from build123d import *

# Parameters (mm, degrees)
IZIM1_R                     = 15
Y_KSEKLIK_EKSTR_ZYON1_DEPTH = 55
IZIM2_R                     = 25
Y_KSEKLIK_EKSTR_ZYON2_DEPTH = 25
IZIM3_R                     = 30
Y_KSEKLIK_EKSTR_ZYON3_DEPTH = 20
IZIM4_W                     = 21.622627276
IZIM4_H                     = 20
KES_EKSTR_ZYON1_DEPTH       = 20
IZIM6_R                     = 4
KES_EKSTR_ZYON2_DEPTH       = 30
KES_EKSTR_ZYON3_DEPTH       = 30


with BuildPart() as part:
    # Çizim1 → Yükseklik-Ekstrüzyon1 (new body)
    with BuildSketch(Plane.XY):
        Circle(IZIM1_R)
    extrude(amount=-Y_KSEKLIK_EKSTR_ZYON1_DEPTH)

    # Çizim2 → Yükseklik-Ekstrüzyon2 (add)
    with BuildSketch(Plane(origin=(0, 0, -55), x_dir=(-1, 0, 0), z_dir=(0, 0, -1))):
        with Locations(Location((0, 10, 0), (0, 0, 270))):
            Circle(IZIM2_R)
    extrude(amount=Y_KSEKLIK_EKSTR_ZYON2_DEPTH)

    # Çizim3 → Yükseklik-Ekstrüzyon3 (add)
    with BuildSketch(Plane(origin=(0, 0, -80), x_dir=(-1, 0, 0), z_dir=(0, 0, -1))):
        with Locations((0, 10)):
            Circle(IZIM3_R)
    extrude(amount=Y_KSEKLIK_EKSTR_ZYON3_DEPTH)

    # Çizim4 → Kes-Ekstrüzyon1 (cut)
    with BuildSketch(Plane(origin=(0, 10, 0), x_dir=(1, 0, 0), z_dir=(0, 1, 0))):
        with Locations((0, 10)):
            Rectangle(IZIM4_W, IZIM4_H)
    extrude(amount=KES_EKSTR_ZYON1_DEPTH, mode=Mode.SUBTRACT)

    # Çizim6 → Kes-Ekstrüzyon2 (cut)
    with BuildSketch(Plane(origin=(0, 10, 0), x_dir=(1, 0, 0), z_dir=(0, 1, 0))):
        with Locations(Location((0, 10, 0), (0, 0, 270))):
            Circle(IZIM6_R)
    extrude(amount=-KES_EKSTR_ZYON2_DEPTH, mode=Mode.SUBTRACT)

    # Çizim7 → Kes-Ekstrüzyon3 (cut)
    with BuildSketch(Plane(origin=(21, 0, 0), x_dir=(0, 0, -1), z_dir=(1, 0, 0))):
        Polygon((55, -7.517008245), (80, -7.517008245), (80, -20), (85, -20), (85, 40), (80, 40), (80, 25), (55, 25), align=None)
    kes_ekstr_zyon3 = extrude(amount=KES_EKSTR_ZYON3_DEPTH, mode=Mode.SUBTRACT)

    # Aynalama1: Kes-Ekstrüzyon3 across plane
    add(kes_ekstr_zyon3.mirror(Plane(origin=(0, 0, 0), x_dir=(0, 0, 1), z_dir=(1, 0, 0))), mode=Mode.SUBTRACT)


solid = part.part
Input: part model. Units: mm. Frame: model coordinates. A direction names the side the tool comes from. Give positions to 0.01 mm unless a question says otherwise; leave off trailing zeros. Order: outer loops, then holes, each group sorted by start corner. A loop starts at its lowest first (then second) coordinate and runs counter-clockwise, first axis right, second up.
Q1. Section B-B on z = -11.5. Output: boundary loops of the cut face in (x, y), and give its area (3 significant figures).
Checked values:
outline: (-10.81, 10) - (-10.81, 10.4) arc R15 ccw to (-3.71, -14.53) - (-3.71, 10) - close; (3.71, -14.53) arc R15 ccw to (10.81, 10.4) - (10.81, 10) - (3.71, 10) - close
area: 445 mm2
Q2. Contact query for flat-ended pins moving along their axis: pin 1 Ø5.5 at (x, y) = (5.5, 13.5) entering from +Z; pin 2 Ø5 at (x, y) = (10, 28) entering from +Z; pin 3 Ø5 at (x, z) = (-13.5, -81.5) entering from +Y; pin 4 Ø6 at (x, z) = (0.5, -10) entering from +Y. Output: stop coordinate, or through.
Checked values:
pin 1: stops at z = -20
pin 2: stops at z = -55
pin 3: stops at y = 37.91
pin 4: passes through
Q3. Set-up query: faces 1 (the cylindrical face through (-3.252, -14.643, -27.115)), 2 (the flat face through (-21, 10, -70)), 3 (the cylindrical face through (0, -15, -67)), 4 (the flat face through (24, 10, -85)). Return all of +Z, -Z, +X, -X, +Y, -Y with unobstructed straight access to the full face (end or side cutting, diameter ignored); none if empty.
Checked values:
face 1: +Z
face 2: +Z, -X, +Y, -Y
face 3: +Z, -Y
face 4: +Z, +X, +Y, -Y
Q4. Section D-D on x = -19. Output: boundary loops of the cut face in (y, z), and give its area (3 significant figures).
Checked values:
outline: (-13.22, -100) - (33.22, -100) - (33.22, -80) - (26.25, -80) - (26.25, -55) - (-6.25, -55) - (-6.25, -80) - (-13.22, -80) - close
area: 1,740 mm2
Q5. Draft query along X for faces 5 (the cylindrical face through (-2.4, -2.3, -13.2)), 6 (the cylindrical face through (0, 35, -67)), 7 (the flat face through (0.1, -15.4, -80)). Return one class per face: +X half, -X half, draft (parallel to the pull), parting line (faces both ways), or undercut.
Checked values:
face 5: undercut
face 6: parting line
face 7: draft
Q6. Section A-A on y = 3.5. Output: boundary loops of the cut face in (x, z).
Checked values:
outline: (-29.29, -100) - (29.29, -100) - (29.29, -85) - (21, -85) - (21, -55) - (14.59, -55) - (14.59, 0) - (-14.59, 0) - (-14.59, -55) - (-21, -55) - (-21, -85) - (-29.29, -85) - close; hole circle Ø8 at (0, -10)
Q7. Section C-C on y = 25. Output: boundary loops of the cut face in (x, z), and give its area (3 significant figures).
Checked values:
outline: (-25.98, -100) - (25.98, -100) - (25.98, -85) - (21, -85) - (21, -80) - (20, -80) - (20, -55) - (-20, -55) - (-20, -80) - (-21, -80) - (-21, -85) - (-25.98, -85) - close
area: 1,990 mm2
Q8. Ray query, probe 1 along X at (y, z) = (0, -10); probe 2 along Z at (x, y) = (0, -0.75); probe 3 along Z at (x, y) = (8, 23.5). Return the intervals inside material, ascending.
Checked values:
probe 1: x = -15 to -4, 4 to 15
probe 2: z = -100 to -14, -6 to 0
probe 3: z = -100 to -55
